Geometry check sheet. Reference: drawing and pictorial views, mm from the part's lowest x, y, z. Give positions to 0.01 mm unless a question says otherwise; leave off trailing zeros. Order: outer loops, then holes, each group sorted by start corner. A loop starts at its lowest first (then second) coordinate and runs counter-clockwise, first axis right, second up.
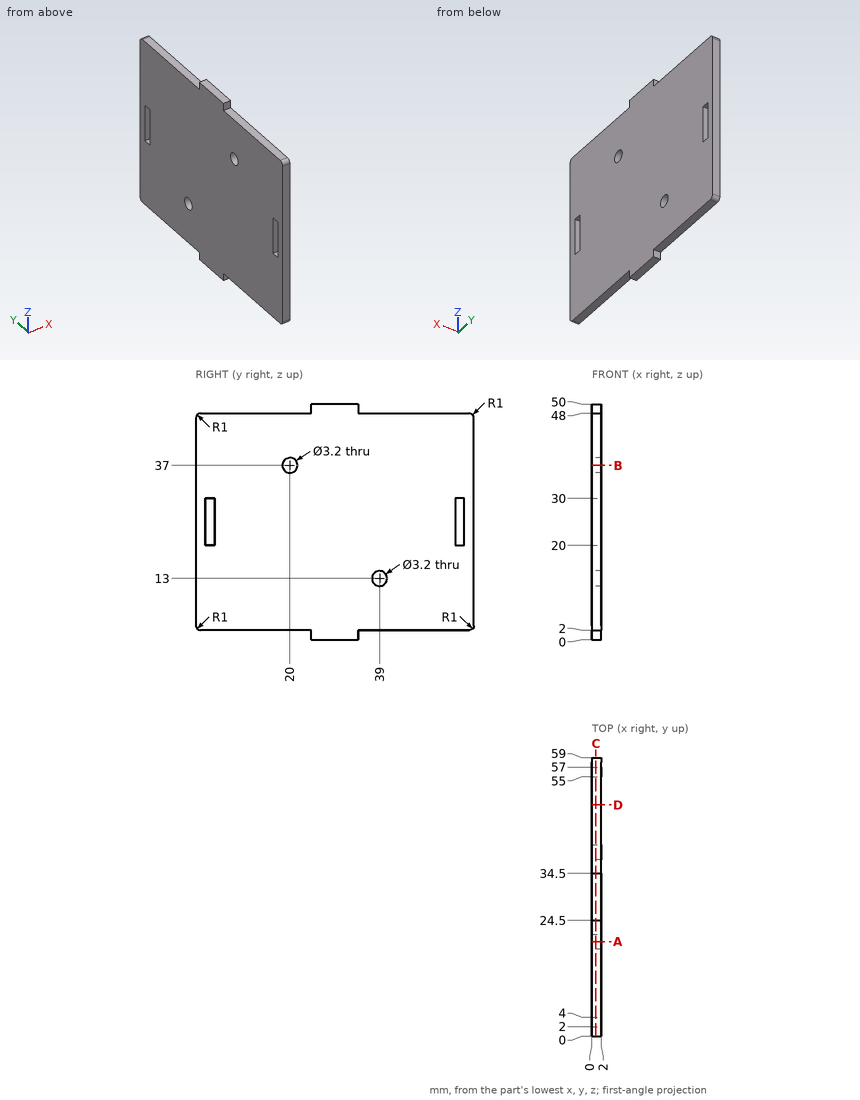
(1) Gauge pin test, flat ends, axial feed: pin 1 Ø1 at (x, y) = (0.5, 45) entering from -Z; pin 2 Ø0.6 at (x, z) = (0.5, 49) entering from -Y; pin 3 Ø1 at (x, y) = (0.5, 3.5) entering from +Z. Record the tip position at first contact, or that the pin passes through.
Response values:
pin 1: stops at z = 2
pin 2: stops at y = 24.5
pin 3: stops at z = 48
(2) Material ranges on L1, parallel to Y at x = 1, z = 23; L2, parallel to Z at x = 0.8, y = 20; L3, parallel to Z at x = 1.7, y = 54.5, recorded low to high.
Response values:
L1: y = 0 to 2, 4 to 55, 57 to 59
L2: z = 2 to 35.4, 38.6 to 48
L3: z = 2 to 48
(3) Cross-section at D-D on y = 49. Enter the section's corners in (x, z), then the cut area to 3 significant figures.
Response values:
outline: (0, 2) - (2, 2) - (2, 48) - (0, 48) - close
area: 92.0 mm2
(4) Cross-section at B-B on z = 37. Enter the section's corners in (x, y).
Response values:
outline: (0, 0) - (2, 0) - (2, 18.4) - (0, 18.4) - close; (0, 21.6) - (2, 21.6) - (2, 59) - (0, 59) - close
(5) Cross-section at C-C on x = 0.85. Enter the section's corners in (y, z).
Response values:
outline: (0, 3) arc R1 ccw to (1, 2) - (24.5, 2) - (24.5, 0) - (34.5, 0) - (34.5, 2) - (58, 2) arc R1 ccw to (59, 3) - (59, 47) arc R1 ccw to (58, 48) - (34.5, 48) - (34.5, 50) - (24.5, 50) - (24.5, 48) - (1, 48) arc R1 ccw to (0, 47) - close; hole (2, 20) - (4, 20) - (4, 30) - (2, 30) - close; hole circle Ø3.2 at (20, 37); hole circle Ø3.2 at (39, 13); hole (55, 20) - (57, 20) - (57, 30) - (55, 30) - close
(6) Cross-section at A-A on y = 20. Enter the section's corners in (x, z).
Response values:
outline: (0, 2) - (2, 2) - (2, 35.4) - (0, 35.4) - close; (0, 38.6) - (2, 38.6) - (2, 48) - (0, 48) - close
